```python
from build123d import *

# Parameters (mm, degrees)
T_LE_DE_BASE_PLI_E1_DEPTH             = 1
T_LE_PLI_E_SUR_AR_TE1_STRIP_W         = 5.4732
T_LE_PLI_E_SUR_AR_TE1_STRIP_H         = 1
T_LE_PLI_E_SUR_AR_TE1_STRIP_CUT_DEPTH = 63.8
T_LE_PLI_E_SUR_AR_TE1_DEPTH           = 63.8
ESQUISSE6_R                           = 2
ESQUISSE6_W                           = 40.8
ESQUISSE6_H                           = 20.9
ENL_V_MAT_EXTRU_1_DEPTH               = 4
ESQUISSE7_R                           = 2
ENL_V_MAT_EXTRU_2_DEPTH               = 63.908187067


# Sheet-metal steps are written as plain solids
with BuildPart() as part:
    # Esquisse1 → Tôle de base pliée1 (new body)
    with BuildSketch(Plane.XY):
        Polygon((-48.8, 10), (0, 30), (15, 30), (15, 0), (-48.8, 0), align=None)
    extrude(amount=T_LE_DE_BASE_PLI_E1_DEPTH)

    # Tôle pliée sur arête1 strip (across the edge) → Tôle pliée sur arête1 strip cut (cut)
    with BuildSketch(Plane(origin=(-48.8, 0, 1), x_dir=(0, 1, 0), z_dir=(1, 0, 0))):
        with Locations((-1, -0.5)):
            Rectangle(T_LE_PLI_E_SUR_AR_TE1_STRIP_W, T_LE_PLI_E_SUR_AR_TE1_STRIP_H)
    extrude(amount=T_LE_PLI_E_SUR_AR_TE1_STRIP_CUT_DEPTH, mode=Mode.SUBTRACT)

    # Tôle pliée sur arête1 section (across the edge) → Tôle pliée sur arête1 (add)
    with BuildSketch(Plane(origin=(-48.8, 0, 1), x_dir=(0, 1, 0), z_dir=(1, 0, 0))):
        with BuildLine():
            Line((0, 0.7366), (0, 26))
            Line((0, 26), (1, 26))
            Line((1, 26), (1, 0.7366))
            ThreePointArc((1, 0.7366), (1.215745145, 0.215745145), (1.7366, 0))
            Line((1.7366, 0), (1.7366, -1))
            ThreePointArc((1.7366, -1), (0.508638364, -0.491361636), (0, 0.7366))
        make_face()
    extrude(amount=T_LE_PLI_E_SUR_AR_TE1_DEPTH)

    # Esquisse6 → Enlèv. mat.-Extru.1 (cut)
    with BuildSketch(Plane.XZ):
        with Locations(Location((3.6, 15.95, 0), (0, 0, 270))):
            Circle(ESQUISSE6_R)
        with Locations(Location((3.6, 5.95, 0), (0, 0, 270))):
            Circle(ESQUISSE6_R)
        with Locations(Location((-44.4, 15.95, 0), (0, 0, 270))):
            Circle(ESQUISSE6_R)
        with Locations(Location((-44.4, 5.95, 0), (0, 0, 270))):
            Circle(ESQUISSE6_R)
        with Locations((-20.4, 10.45)):
            Rectangle(ESQUISSE6_W, ESQUISSE6_H)
    extrude(amount=-ENL_V_MAT_EXTRU_1_DEPTH, mode=Mode.SUBTRACT)

    # Esquisse7 → Enlèv. mat.-Extru.2 (cut, through all)
    with BuildSketch(Plane.XY.offset(1)):
        with Locations((7.5, 22)):
            Circle(ESQUISSE7_R)
        with Locations((7.5, 6)):
            Circle(ESQUISSE7_R)
    extrude(amount=-ENL_V_MAT_EXTRU_2_DEPTH, mode=Mode.SUBTRACT)


solid = part.part
```
Build history of the part. All positions in model axes, mm. A direction names the side the tool comes from. Coordinates: 2 decimals unless noted, no trailing zeros. Order: outer loops, then holes, each group sorted by start corner. A loop starts at its lowest first (then second) coordinate and runs counter-clockwise, first axis right, second up. Notation, with made-up numbers: (21.5, 51) -> (52.5, 51) arc R9 cw to (52.5, 60) -> close; hole circle Ø6 at (72.5, 75). An arc over 180 degrees is marked (long way). Answer in a Markdown table with one row per item. Add a question column.
Q1. Band-saw the part on C-C, the plane z = 16.25. List the corners of the cut face in (x, y).
Q2. Band-saw the part on D-D, the plane x = -12.5. List the corners of the cut face in (y, z).
Q3. Band-saw the part on A-A, the plane x = 3.6. List the corners of the cut face in (y, z).
Q4. Wall check: line 1 along X through (y, z) = (0.5, 5.95); line 2 along Y through (x, z) = (7.5, 0.45); line 3 along Y through (x, z) = (7.5, 0.7). Give the ranges that are in metal, low to high. Write a range as [from, to].
Q5. Band-saw the part on B-B, the plane y = 22. List the corners of the cut face in (x, z), then the cut area to 3 significant figures.
Q6. Drop flat-ended pins along their axis: pin 1 (6 mm diameter, centred on x = -14, y = 19.5, fed in from +Z); pin 2 (1.1 mm diameter, centred on x = -17, y = 0.5, fed in from -Z). Give the stop position or say it passes through.
Q7. Which spindle directions (+Z, -Z, +X, -X, +Y, -Y) get a long thin tool onto all of the face, cutting with end or side? Do faces 1 (the face through (-9, 16, 0)), 2 (the face through (-10, 1, 23)). Say none if no direction does.
Q8. Mould opens along Y. For faces 3 (the face through (-24.74, 19.86, 0.49)), 4 (the face through (7.39, 0.52, 0.5)), 5 (the face through (5.502, 6.088, 0.507)), 6 (the face through (-45.617, 0.493, 17.537)) say: +Y half, -Y half, draft (parallel to the pull), parting line (faces both ways), or undercut.
Answers follow:
| question | item | result |
|---|---|---|
| 1 | outline | (-48.8, 0) -> (-46.38, 0) -> (-46.38, 1) -> (-48.8, 1) -> close; (-42.42, 0) -> (-40.8, 0) -> (-40.8, 1) -> (-42.42, 1) -> close; (0, 0) -> (1.62, 0) -> (1.62, 1) -> (0, 1) -> close; (5.58, 0) -> (15, 0) -> (15, 1) -> (5.58, 1) -> close |
| 2 | outline | (0, 20.9) -> (1, 20.9) -> (1, 27) -> (0, 27) -> close; (4, 0) -> (24.88, 0) -> (24.88, 1) -> (4, 1) -> close |
| 3 | outline | (0, 1.74) arc R1.74 ccw to (1.74, 0) -> (30, 0) -> (30, 1) -> (1.74, 1) arc R0.74 cw to (1, 1.74) -> (1, 3.95) -> (0, 3.95) -> close; (0, 7.95) -> (1, 7.95) -> (1, 13.95) -> (0, 13.95) -> close; (0, 17.95) -> (1, 17.95) -> (1, 27) -> (0, 27) -> close |
| 4 | line 1 | [-48.8, -46.4], [-42.4, -40.8], [0, 1.6], [5.6, 15] |
| 4 | line 2 | [0.57, 4], [8, 20], [24, 30] |
| 4 | line 3 | [0.34, 4], [8, 20], [24, 30] |
| 5 | outline | (-19.52, 0) -> (5.5, 0) -> (5.5, 1) -> (-19.52, 1) -> close; (9.5, 0) -> (15, 0) -> (15, 1) -> (9.5, 1) -> close |
| 5 | area | 30.5 mm^2 |
| 6 | pin 1 | z = 1 |
| 6 | pin 2 | z = 20.9 |
| 7 | face 1 | -Z, +X, -X, +Y, -Y |
| 7 | face 2 | +Z, +X, -X, +Y |
| 8 | face 3 | +Y half |
| 8 | face 4 | -Y half |
| 8 | face 5 | undercut |
| 8 | face 6 | draft |
